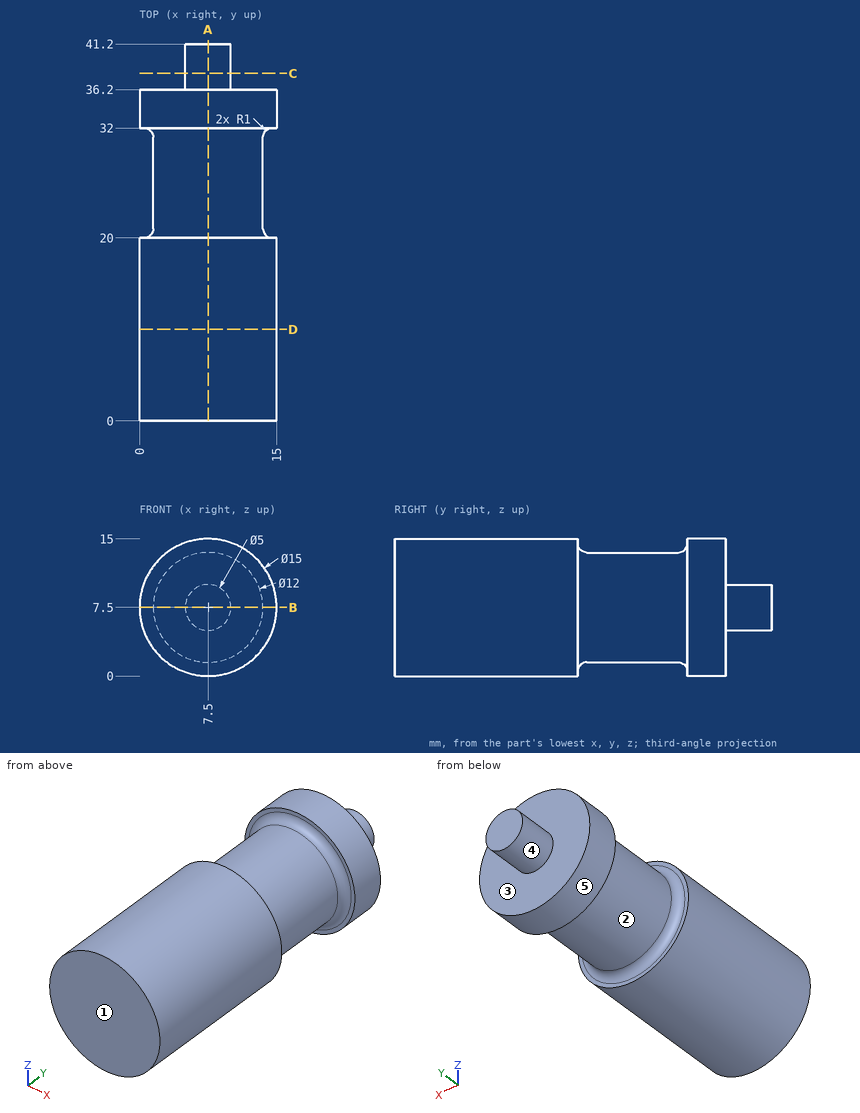
Geometry check sheet. Reference: drawing and pictorial views, mm from the part's lowest x, y, z. A direction names the side the tool comes from. Give positions to 0.01 mm unless a question says otherwise; leave off trailing zeros. Write each loop counter-clockwise with the first axis right and the second up, starting at its lowest first coordinate (ties: lowest second). Pieces come first, ordered by that corner, then holes. Notation, with made-up numbers: M 29,17.25 L 71,17.25 A22 ccw 71,33.25 Z; hole C 51,65 d7. An arc over 180 degrees is marked long. Use CSV: the item, a comma, the result in double quotes.
1) Release check for a two-part mould opening along Y. For the marked faces 1, 2 and 3 record: released by +Y, released by -Y, zero draft, split by the parting line, or undercut.
Final values:
face 1,"released by -Y"
face 2,"undercut"
face 3,"released by +Y"
2) Cross-section at A-A (x = 7.5). Enter the section's corners in (y, z), plus the area to 3 significant figures.
Final values:
outline,"M 0,0 L 20,0 L 20,0.5 A1 cw 21,1.5 L 31,1.5 A1 cw 32,0.5 L 32,0 L 36.2,0 L 36.2,5 L 41.2,5 L 41.2,10 L 36.2,10 L 36.2,15 L 32,15 L 32,14.5 A1 cw 31,13.5 L 21,13.5 A1 cw 20,14.5 L 20,15 L 0,15 Z"
area,"533 mm²"
3) Cross-section at C-C (y = 38). Enter the section's corners in (x, z).
Final values:
outline,"C 7.5,7.5 d5"
4) Cross-section at B-B (z = 7.5). Enter the section's corners in (x, y), plus the area to 3 significant figures.
Final values:
outline,"M 0,0 L 15,0 L 15,20 L 14.5,20 A1 cw 13.5,21 L 13.5,31 A1 cw 14.5,32 L 15,32 L 15,36.2 L 10,36.2 L 10,41.2 L 5,41.2 L 5,36.2 L 0,36.2 L 0,32 L 0.5,32 A1 cw 1.5,31 L 1.5,21 A1 cw 0.5,20 L 0,20 Z"
area,"533 mm²"
5) Material ranges on line 1 along Y through (x, z) = (8.75, 14.25); line 2 along Z through (x, y) = (3, 13); line 3 along Y through (x, z) = (8, 1.25), recorded low to high.
Final values:
line 1,"0 to 20.01, 31.99 to 36.2"
line 2,"1.5 to 13.5"
line 3,"0 to 20.32, 31.68 to 36.2"
6) Access from +Z, -Z, +X, -X, +Y, -Y to the whole of each face (thin tool, end or side, straight path). Record for the marked faces 4 and 5.
Final values:
face 4,"+Y"
face 5,"+Y, -Y"
7) Cross-section at D-D (y = 10). Enter the section's corners in (x, z), plus the area to 3 significant figures.
Final values:
outline,"C 7.5,7.5 d15"
area,"177 mm²"
8) Go/stop test with flat-tipped pins: pin 1 Ø5 at (x, y) = (2, 31) entering from +Z; pin 2 Ø4 at (y, z) = (27.5, 5) entering from +X; pin 3 Ø4.5 at (x, z) = (4, 4) entering from +Y; pin 4 Ø1 at (x, z) = (2, 1.5) entering from -Y. Record where each tip stops, or that it passes through.
Final values:
pin 1,"z = 14.28"
pin 2,"x = 13.48"
pin 3,"y = 36.2"
pin 4,"through"
